from build123d import *

# Parameters (mm, degrees)
BOSS_EXTRUDE1_DEPTH = 18
CUT_EXTRUDE1_REACH  = 4
SKETCH2_R           = 2
CUT_EXTRUDE2_REACH  = 4
SKETCH3_R           = 2


with BuildPart() as part:
    # Sketch1 → Boss-Extrude1 (new body)
    with BuildSketch(Plane.XY):
        Polygon((0, 0), (100, 0), (100, 11), (128, 11), (128, 9), (102, 9), (102, -2), (0, -2), align=None)
    extrude(amount=BOSS_EXTRUDE1_DEPTH)

    # Sketch2 → Cut-Extrude1 (cut, up to next)
    with BuildSketch(Plane(origin=(0, 0, 0), x_dir=(1, 0, 0), z_dir=(0, 1, 0)), mode=Mode.PRIVATE) as cut_extrude1_sk1:
        with Locations((4, -14)):
            Circle(SKETCH2_R)
    cut_extrude1_tool1 = extrude(cut_extrude1_sk1.sketch, amount=-CUT_EXTRUDE1_REACH, mode=Mode.PRIVATE) & part.part
    add(cut_extrude1_tool1.solids().sort_by_distance((4, 0, 14))[0], mode=Mode.SUBTRACT)
    # Sketch2 → Cut-Extrude1 (cut, up to next)
    with BuildSketch(Plane(origin=(0, 0, 0), x_dir=(1, 0, 0), z_dir=(0, 1, 0)), mode=Mode.PRIVATE) as cut_extrude1_sk2:
        with Locations((4, -4)):
            Circle(SKETCH2_R)
    cut_extrude1_tool2 = extrude(cut_extrude1_sk2.sketch, amount=-CUT_EXTRUDE1_REACH, mode=Mode.PRIVATE) & part.part
    add(cut_extrude1_tool2.solids().sort_by_distance((4, 0, 4))[0], mode=Mode.SUBTRACT)
    # Sketch2 → Cut-Extrude1 (cut, up to next)
    with BuildSketch(Plane(origin=(0, 0, 0), x_dir=(1, 0, 0), z_dir=(0, 1, 0)), mode=Mode.PRIVATE) as cut_extrude1_sk3:
        with Locations((26, -14)):
            Circle(SKETCH2_R)
    cut_extrude1_tool3 = extrude(cut_extrude1_sk3.sketch, amount=-CUT_EXTRUDE1_REACH, mode=Mode.PRIVATE) & part.part
    add(cut_extrude1_tool3.solids().sort_by_distance((26, 0, 14))[0], mode=Mode.SUBTRACT)
    # Sketch2 → Cut-Extrude1 (cut, up to next)
    with BuildSketch(Plane(origin=(0, 0, 0), x_dir=(1, 0, 0), z_dir=(0, 1, 0)), mode=Mode.PRIVATE) as cut_extrude1_sk4:
        with Locations((26, -4)):
            Circle(SKETCH2_R)
    cut_extrude1_tool4 = extrude(cut_extrude1_sk4.sketch, amount=-CUT_EXTRUDE1_REACH, mode=Mode.PRIVATE) & part.part
    add(cut_extrude1_tool4.solids().sort_by_distance((26, 0, 4))[0], mode=Mode.SUBTRACT)

    # Sketch3 → Cut-Extrude2 (cut, up to next)
    with BuildSketch(Plane.XZ.offset(-9), mode=Mode.PRIVATE) as cut_extrude2_sk1:
        with Locations((120, 9)):
            Circle(SKETCH3_R)
    cut_extrude2_tool1 = extrude(cut_extrude2_sk1.sketch, amount=-CUT_EXTRUDE2_REACH, mode=Mode.PRIVATE) & part.part
    add(cut_extrude2_tool1.solids().sort_by_distance((120, 9, 9))[0], mode=Mode.SUBTRACT)
    # Sketch3 → Cut-Extrude2 (cut, up to next)
    with BuildSketch(Plane.XZ.offset(-9), mode=Mode.PRIVATE) as cut_extrude2_sk2:
        with Locations((110, 9)):
            Circle(SKETCH3_R)
    cut_extrude2_tool2 = extrude(cut_extrude2_sk2.sketch, amount=-CUT_EXTRUDE2_REACH, mode=Mode.PRIVATE) & part.part
    add(cut_extrude2_tool2.solids().sort_by_distance((110, 9, 9))[0], mode=Mode.SUBTRACT)


solid = part.part
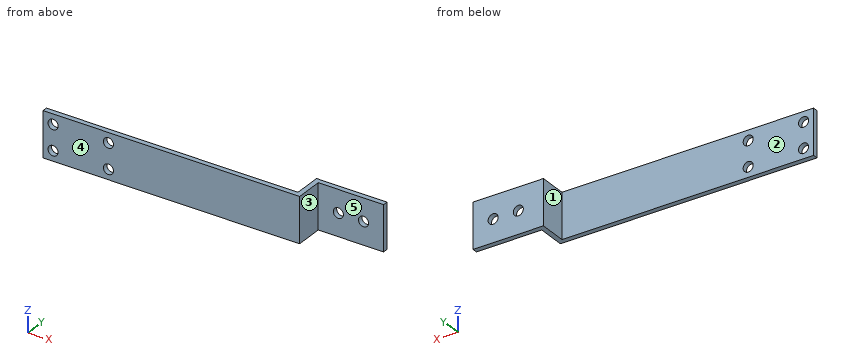
Design review of the part built by this model. Coordinates are the model's own, in mm. Face numbers are marked on the shaded views. A direction names the side the tool comes from. Round coordinates to 2 decimals unless told otherwise and drop trailing zeros. Write each loop counter-clockwise with the first axis right and the second up, starting at its lowest first coordinate (ties: lowest second). Pieces come first, ordered by that corner, then holes.
Item 1: Wall thickness on L1, parallel to X at y = -1.6, z = 4; L2, parallel to Z at x = 4, y = -0.65; L3, parallel to Z at x = 110, y = 9.45: over which ranges is each line inside the solid? List them lowest first.
Item 2: Consider section C-C on x = 120. Give the boundary of the cut face in (y, z).
Item 3: For pin 1 Ø2 at (y, z) = (7.5, 2.5) entering from +X; pin 2 Ø1 at (x, z) = (28.5, 2.5) entering from +Y; pin 3 Ø1 at (x, z) = (25, 3) entering from +Y; pin 4 Ø9 at (x, z) = (117.5, 13) entering from -Y, all flat-tipped, find the tip position at first contact; note any pin that passes through.
Item 4: Draft analysis for pull direction X (two halves, no side actions). For the marked faces 1, 2 and 3, state which applies: released by +X, released by -X, zero draft, split by the parting line, or undercut.
Item 5: Consider section D-D on y = 3.75. Give the boundary of the cut face in (x, z), and give its area (3 significant figures).
Item 6: Consider section A-A on x = 4. Give the boundary of the cut face in (y, z).
Item 7: Consider section B-B on z = 14. Give the boundary of the cut face in (x, y).
Item 8: For the marked faces 4 and 5, list the 3-axis set-ups (+Z, -Z, +X, -X, +Y, -Y) from which the entire face can be reached by the end or side of a thin tool; tool diameter is ignored.
Check values:
1. L1: x = 0 to 2, 6 to 24, 28 to 102
1. L2: z = 0 to 2, 6 to 12, 16 to 18
1. L3: z = 0 to 7, 11 to 18
2. outline: (9, 0) - (11, 0) - (11, 7) - (9, 7) - close; (9, 11) - (11, 11) - (11, 18) - (9, 18) - close
3. pin 1: stops at x = 102
3. pin 2: stops at y = 0
3. pin 3: passes through
3. pin 4: stops at y = 9
4. face 1: released by -X
4. face 2: zero draft
4. face 3: released by +X
5. outline: (100, 0) - (102, 0) - (102, 18) - (100, 18) - close
5. area: 36.0 mm2
6. outline: (-2, 0) - (0, 0) - (0, 2) - (-2, 2) - close; (-2, 6) - (0, 6) - (0, 12) - (-2, 12) - close; (-2, 16) - (0, 16) - (0, 18) - (-2, 18) - close
7. outline: (0, -2) - (2, -2) - (2, 0) - (0, 0) - close; (6, -2) - (24, -2) - (24, 0) - (6, 0) - close; (28, -2) - (102, -2) - (102, 9) - (128, 9) - (128, 11) - (100, 11) - (100, 0) - (28, 0) - close
8. face 4: +Z, -Z, +X, -X, -Y
8. face 5: +Z, -Z, +X, -Y
